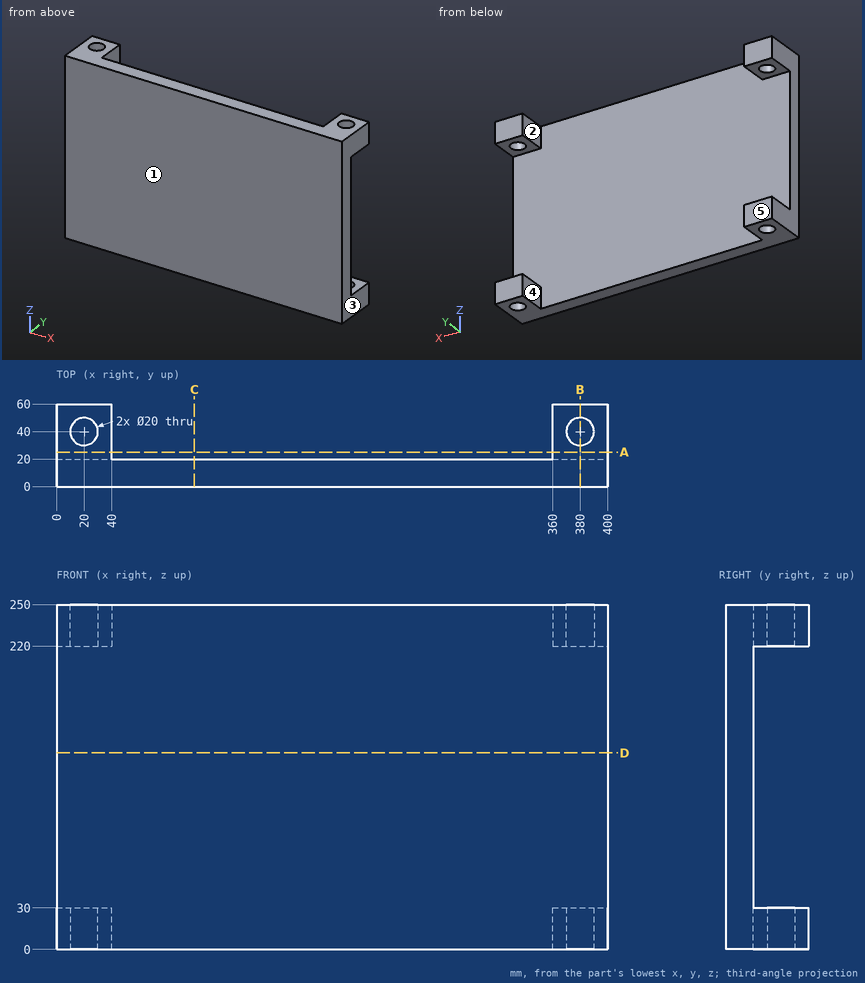
Design review of the part shown in the three views and the two pictorial views. Dimensions are in mm from the part's minimum x, y and z. A direction names the side the tool comes from. Give positions to 0.01 mm unless a question says otherwise; leave off trailing zeros. Loops run counter-clockwise (first coordinate to the right, second up) from the corner with the lowest first, then second, coordinate; pieces in that order, holes last. Notation, with made-up numbers: (-12, 57.25) -> (17, 57.25) arc R32 ccw to (17, 93.25) -> close; hole circle Ø8 at (9, 83). An arc over 180 degrees is marked (long way). One line per question, with ' | ' between items.
1) For the marked faces 1 and 2, list the 3-axis set-ups (+Z, -Z, +X, -X, +Y, -Y) from which the entire face can be reached by the end or side of a thin tool; tool diameter is ignored.
Resolved:
face 1: +Z, -Z, +X, -X, -Y | face 2: +Z, -Z, +Y
2) Insertion check: pin 1 Ø8 at (x, z) = (157, 192.5) entering from +Y. The pin has a flat end and moves straight along its axis. Give the tip position at first contact, or say it passes through.
Resolved:
pin 1: stops at y = 20
3) We need section B-B (x = 380). Write out the cut boundary in (y, z), plus the area to 3 significant figures.
Resolved:
outline: (0, 0) -> (30, 0) -> (30, 30) -> (20, 30) -> (20, 220) -> (30, 220) -> (30, 250) -> (0, 250) -> close; (50, 0) -> (60, 0) -> (60, 30) -> (50, 30) -> close; (50, 220) -> (60, 220) -> (60, 250) -> (50, 250) -> close | area: 6,200 mm2
4) We need section C-C (x = 100). Write out the cut boundary in (y, z).
Resolved:
outline: (0, 0) -> (20, 0) -> (20, 250) -> (0, 250) -> close
5) We need section A-A (y = 25). Write out the cut boundary in (x, z), plus the area to 3 significant figures.
Resolved:
outline: (0, 0) -> (40, 0) -> (40, 30) -> (0, 30) -> close; (0, 220) -> (40, 220) -> (40, 250) -> (0, 250) -> close; (360, 0) -> (400, 0) -> (400, 30) -> (360, 30) -> close; (360, 220) -> (400, 220) -> (400, 250) -> (360, 250) -> close | area: 4,800 mm2
6) We need section D-D (z = 142.5). Write out the cut boundary in (x, y).
Resolved:
outline: (0, 0) -> (400, 0) -> (400, 20) -> (0, 20) -> close
7) The part is to be moulded in two halves that separate along X. For the marked faces 3, 4 and 5, say which applies: +X half, -X half, draft (parallel to the pull), parting line (faces both ways), or undercut.
Resolved:
face 3: +X half | face 4: undercut | face 5: draft
8) To check wall thickness, follow probe 1 along Y at (x, z) = (20, 232); probe 2 along X at (y, z) = (27, 233); probe 3 along X at (y, z) = (39, 18). State the ranges of each line that lie inside material, in increasing order.
Resolved:
probe 1: y = 0 to 30, 50 to 60 | probe 2: x = 0 to 40, 360 to 400 | probe 3: x = 0 to 10.05, 29.95 to 40, 360 to 370.05, 389.95 to 400
